Build history of the part. All positions in model axes, mm. Coordinates: 2 decimals unless noted, no trailing zeros. Loops run counter-clockwise (first coordinate to the right, second up) from the corner with the lowest first, then second, coordinate; pieces in that order, holes last. Notation, with made-up numbers: (73, -25) -> (128, -25) arc R11 cw to (128, -12) -> close; hole circle Ø5 at (77, 85). An arc over 180 degrees is marked (long way). One line per item, written item: value. Start each with the question number.
```python
from build123d import *

# Parameters (mm, degrees)
SKETCH1_W           = 278
SKETCH1_H           = 278
BOSS_EXTRUDE1_DEPTH = 6.35
SKETCH2_R           = 35
SKETCH2_R_2         = 2.75
CUT_EXTRUDE1_DEPTH  = 7.35
CHAMFER1_SIZE       = 20
SKETCH4_R           = 2.75
CUT_EXTRUDE2_DEPTH  = 76.2


with BuildPart() as part:
    # Sketch1 → Boss-Extrude1 (new body)
    with BuildSketch(Plane.XY):
        Rectangle(SKETCH1_W, SKETCH1_H)
    extrude(amount=BOSS_EXTRUDE1_DEPTH)

    # Sketch2 → Cut-Extrude1 (cut, through all)
    with BuildSketch(Plane.XY.offset(6.35)):
        Circle(SKETCH2_R)
        with Locations((-40, 40)):
            Circle(SKETCH2_R_2)
        with Locations((40, 40)):
            Circle(SKETCH2_R_2)
        with Locations((40, -40)):
            Circle(SKETCH2_R_2)
        with Locations((-40, -40)):
            Circle(SKETCH2_R_2)
    extrude(amount=-CUT_EXTRUDE1_DEPTH, mode=Mode.SUBTRACT)

    # Chamfer1
    chamfer1_edges = [part.edges().sort_by_distance(p)[0] for p in [
        (-139, 139, 3.175),
        (139, 139, 3.175),
        (139, -139, 3.175),
        (-139, -139, 3.175),
    ]]
    chamfer(chamfer1_edges, length=CHAMFER1_SIZE)

    # Sketch4 → Cut-Extrude2 (cut)
    with BuildSketch(Plane.XY.offset(6.35)):
        with Locations((-90, 130)):
            Circle(SKETCH4_R)
        with Locations((0, 130)):
            Circle(SKETCH4_R)
        with Locations((90, 130)):
            Circle(SKETCH4_R)
        with Locations((90, -130)):
            Circle(SKETCH4_R)
        with Locations((0, -130)):
            Circle(SKETCH4_R)
        with Locations((-90, -130)):
            Circle(SKETCH4_R)
    extrude(amount=-CUT_EXTRUDE2_DEPTH, mode=Mode.SUBTRACT)


solid = part.part
```
Item 1: Probe probe 1 along Y at (x, z) = (40, 4); probe 2 along Y at (x, z) = (-90, 1.75); probe 3 along X at (y, z) = (-2, 1.5). List the from-to ranges inside material, lowest first.
Item 2: Two-plate mould, pull along Y, no slides. Class faces 1 (the face through (139, -2, 3)), 2 (the face through (-129, -129, 3)), 3 (the face through (-28, -21, 3)): +Y half, -Y half, draft (parallel to the pull), parting line (faces both ways), or undercut.
Item 3: Drop a flat-ended pin along its axis: pin 1 Ø6.5 at (x, y) = (-40, -40) entering from -Z. Give the stop position or say it passes through.
Item 4: Band-saw the part on A-A, the plane y = 0. List the corners of the cut face in (x, z).
Item 5: Band-saw the part on B-B, the plane z = 3.75. Count the separate pieces of the cut face and the enclosed holes in it, and give its area (3 significant figures).
Item 6: Band-saw the part on C-C, the plane x = -25.5. List the corners of the cut face in (y, z).
Worked out:
1. probe 1: y = -139 to -42.75, -37.25 to 37.25, 42.75 to 139
1. probe 2: y = -139 to -132.75, -127.25 to 127.25, 132.75 to 139
1. probe 3: x = -139 to -34.94, 34.94 to 139
2. face 1: draft
2. face 2: -Y half
2. face 3: undercut
3. pin 1: stops at z = 0
4. outline: (-139, 0) -> (-35, 0) -> (-35, 6.35) -> (-139, 6.35) -> close; (35, 0) -> (139, 0) -> (139, 6.35) -> (35, 6.35) -> close
5. separate pieces: 1
5. enclosed holes: 11
5. area: 72,400 mm²
6. outline: (-139, 0) -> (-23.97, 0) -> (-23.97, 6.35) -> (-139, 6.35) -> close; (23.97, 0) -> (139, 0) -> (139, 6.35) -> (23.97, 6.35) -> close
